Can you work these out from the model? Positions are in its coordinate system, mm. A direction names the side the tool comes from. Coordinates: 2 decimals unless noted, no trailing zeros. Loops run counter-clockwise (first coordinate to the right, second up) from the corner with the lowest first, then second, coordinate; pieces in that order, holes last. Notation, with made-up numbers: M 43.25,71 L 57.25,71 A24 ccw 57.25,97 Z; hole C -11.75,71 d6. An arc over 180 degrees is marked long. Answer as a JSON object with one key per item and string values. Group by question number.
Item 1: Suppose I cut it at A-A (y = 12.25). Write out the boundary of the cut face in (x, z) (3 decimals).
Item 2: Suppose I cut it at C-C (x = -9.5). Write out the boundary of the cut face in (y, z) (3 decimals).
Item 3: I'm going to push flat-ended pins straight in: pin 1 Ø2 at (x, z) = (28.5, -14) entering from +Y; pin 2 Ø1.3 at (x, y) = (-54, 0.5) entering from +Z; pin 3 Ø3 at (y, z) = (12.5, -34.5) entering from +X (3 decimals); pin 4 Ø1.9 at (x, z) = (-36, -43) entering from +Y (3 decimals). Where does each tip first touch, or does it pass through?
Item 4: Suppose I cut it at D-D (x = -50). Write out the boundary of the cut face in (y, z).
Item 5: Which directions (+Z, -Z, +X, -X, +Y, -Y) give clear straight access to the entire face, cutting with the end or side of a thin tool? Please do faces 1 (the flat face through (39.305, 9, 30)), 2 (the flat face through (-40, 15.92, 3)), 3 (the flat face through (42, 9, -28.515)), 4 (the flat face through (-39, 1.59, 41)).
Item 6: If I drill on line 1 (X direction, y = 1.75, z = 2.5) (3 decimals); line 2 (Y direction, x = 48, z = -6.5); line 3 (Z direction, x = 44, y = 6) (3 decimals), over which ranges is the centre line in solid material (lowest first)?
Item 7: We'd pull the mould along X, two halves only. Please class faces 5 (the flat face through (-44.385, 9, 2)), 6 (the cylindrical face through (39.527, 0.796, 44.382)), 7 (the flat face through (1, 1.57, -1)), 8 (the flat face through (36, 1.59, -44)): +X half, -X half, draft (parallel to the pull), parting line (faces both ways), or undercut.
Item 8: Suppose I cut it at B-B (z = 2). Write out the boundary of the cut face in (x, y) (3 decimals).
```python
from build123d import *

# Parameters (mm, degrees)
BASE_EXTRUDE_DEPTH   = 1.57
SKETCH2_R            = 1.59
MOUNTING_HOLES_DEPTH = 76.101891787
SKETCH3_R            = 3.175
SKETCH3_R_2          = 1.59
TOP_PADS_DEPTH       = 0.02
SKETCH4_R            = 3.175
SKETCH4_R_2          = 1.59
BOTT_PADS_DEPTH      = 0.02
ISA_CNCT_DEPTH       = 16.05
SKETCH6_W            = 8
SKETCH6_H            = 60.3
PCI_CNCT_DEPTH       = 14.35


with BuildPart() as part:
    # Sketch1 → Base-Extrude (new body)
    with BuildSketch(Plane(origin=(0, 0, 0), x_dir=(1, 0, 0), z_dir=(0, 1, 0))):
        Polygon((-45.085, 47.945), (45.085, 47.945), (45.085, 40.343374485), (57.785, 40.343374485), (57.785, -40.318146652), (45.085, -40.318146652), (45.085, -47.945), (-45.085, -47.945), (-45.085, -40.318146652), (-57.785, -40.318146652), (-57.785, 40.343374485), (-45.085, 40.343374485), align=None)
    extrude(amount=BASE_EXTRUDE_DEPTH)

    # Sketch2 → Mounting Holes (cut, through all)
    with BuildSketch(Plane(origin=(0, 1.57, 0), x_dir=(-1, 0, 0), z_dir=(0, 1, 0))):
        with Locations(Location((36.195, -42.865, 0), (0, 0, 90))):
            Circle(SKETCH2_R)
        with Locations(Location((40.005, 42.865, 0), (0, 0, 90))):
            Circle(SKETCH2_R)
        with Locations(Location((-40.005, 42.865, 0), (0, 0, 90))):
            Circle(SKETCH2_R)
        with Locations(Location((-37.465, -42.865, 0), (0, 0, 90))):
            Circle(SKETCH2_R)
    extrude(amount=-MOUNTING_HOLES_DEPTH, mode=Mode.SUBTRACT)

    # Sketch3 → Top Pads (add)
    with BuildSketch(Plane(origin=(0, 1.57, 0), x_dir=(-1, 0, 0), z_dir=(0, 1, 0))):
        with Locations(Location((36.195, -42.865, 0), (0, 0, 270))):
            Circle(SKETCH3_R)
        with Locations(Location((36.195, -42.865, 0), (0, 0, 90))):
            Circle(SKETCH3_R_2, mode=Mode.SUBTRACT)
        with Locations(Location((-37.465, -42.865, 0), (0, 0, 270))):
            Circle(SKETCH3_R)
        with Locations(Location((-37.465, -42.865, 0), (0, 0, 90))):
            Circle(SKETCH3_R_2, mode=Mode.SUBTRACT)
        with Locations(Location((-40.005, 42.865, 0), (0, 0, 270))):
            Circle(SKETCH3_R)
        with Locations(Location((-40.005, 42.865, 0), (0, 0, 90))):
            Circle(SKETCH3_R_2, mode=Mode.SUBTRACT)
        with Locations(Location((40.005, 42.865, 0), (0, 0, 270))):
            Circle(SKETCH3_R)
        with Locations(Location((40.005, 42.865, 0), (0, 0, 90))):
            Circle(SKETCH3_R_2, mode=Mode.SUBTRACT)
    extrude(amount=TOP_PADS_DEPTH)

    # Sketch4 → Bott Pads (add)
    with BuildSketch(Plane.XZ):
        with Locations(Location((-36.195, -42.865, 0), (0, 0, 270))):
            Circle(SKETCH4_R)
        with Locations(Location((-36.195, -42.865, 0), (0, 0, 90))):
            Circle(SKETCH4_R_2, mode=Mode.SUBTRACT)
        with Locations(Location((37.465, -42.865, 0), (0, 0, 270))):
            Circle(SKETCH4_R)
        with Locations(Location((37.465, -42.865, 0), (0, 0, 90))):
            Circle(SKETCH4_R_2, mode=Mode.SUBTRACT)
        with Locations(Location((40.005, 42.865, 0), (0, 0, 270))):
            Circle(SKETCH4_R)
        with Locations(Location((40.005, 42.865, 0), (0, 0, 90))):
            Circle(SKETCH4_R_2, mode=Mode.SUBTRACT)
        with Locations(Location((-40.005, 42.865, 0), (0, 0, 270))):
            Circle(SKETCH4_R)
        with Locations(Location((-40.005, 42.865, 0), (0, 0, 90))):
            Circle(SKETCH4_R_2, mode=Mode.SUBTRACT)
    extrude(amount=BOTT_PADS_DEPTH)

    # Sketch5 → ISA Cnct (add)
    with BuildSketch(Plane(origin=(0, 1.57, 0), x_dir=(-1, 0, 0), z_dir=(0, 1, 0))):
        Polygon((-39.305, 22.795), (-39.305, 38.115), (-34.355, 38.115), (-34.355, -38.675), (-39.305, -38.675), (-39.305, -28.515), (-44.385, -28.515), (-44.385, 22.795), align=None)
    extrude(amount=ISA_CNCT_DEPTH)

    # Sketch6 → PCI Cnct (add)
    with BuildSketch(Plane(origin=(0, 1.57, 0), x_dir=(-1, 0, 0), z_dir=(0, 1, 0))):
        with Locations((40.385, 2.805)):
            Rectangle(SKETCH6_W, SKETCH6_H)
    extrude(amount=PCI_CNCT_DEPTH)


solid = part.part
```
From the geometry:
{
 "1": {"outline": "M -44.385,-27.345 L -36.385,-27.345 L -36.385,32.955 L -44.385,32.955 Z; M 34.355,-38.675 L 39.305,-38.675 L 39.305,-28.515 L 44.385,-28.515 L 44.385,22.795 L 39.305,22.795 L 39.305,38.115 L 34.355,38.115 Z"},
 "2": {"outline": "M 0,-47.945 L 1.57,-47.945 L 1.57,47.945 L 0,47.945 Z"},
 "3": {"pin 1": "y = 1.57", "pin 2": "z = 40.32", "pin 3": "x = 39.305", "pin 4": "through"},
 "4": {"outline": "M 0,-40.34 L 1.57,-40.34 L 1.57,40.32 L 0,40.32 Z"},
 "5": {"face 1": "+Z, +X, +Y", "face 2": "+Z, -Z, -X, +Y", "face 3": "-Z, +X, +Y", "face 4": "+Z, +X, -X, +Y"},
 "6": {"line 1": "-44.385 to -36.385, 34.355 to 44.385", "line 2": "0 to 1.57", "line 3": "-28.515 to 22.795"},
 "7": {"face 5": "-X half", "face 6": "undercut", "face 7": "undercut", "face 8": "draft"},
 "8": {"outline": "M -57.785,0 L 57.785,0 L 57.785,1.57 L 44.385,1.57 L 44.385,17.62 L 34.355,17.62 L 34.355,1.57 L -36.385,1.57 L -36.385,15.92 L -44.385,15.92 L -44.385,1.57 L -57.785,1.57 Z"}
}
